The model under review builds one solid part; all positions refer to its coordinate system, in mm. Give positions to 0.01 mm unless a question says otherwise; leave off trailing zeros. Return JSON: item names as keys, results as strings. Group by question number.
from build123d import *

# Parameters (mm, degrees)
SKETCH1_W                      = 12
SKETCH1_H                      = 8
BOSS_EXTRUDE1_DEPTH            = 450
CBORE_FOR_M3_SHCS1_D           = 3.4
CBORE_FOR_M3_SHCS1_CBORE_D     = 6.5
CBORE_FOR_M3_SHCS1_CBORE_DEPTH = 4.5


with BuildPart() as part:
    # Sketch1 → Boss-Extrude1 (new body)
    with BuildSketch(Plane.XY):
        with Locations((6, 4)):
            Rectangle(SKETCH1_W, SKETCH1_H)
    extrude(amount=BOSS_EXTRUDE1_DEPTH)

    # CBORE for M3 SHCS1 (through all)
    with Locations(Plane(origin=(0, 8, 0), x_dir=(1, 0, 0), z_dir=(0, 1, 0))):
        with Locations((6, -440), (6, -415), (6, -390), (6, -365), (6, -340), (6, -315), (6, -290), (6, -265), (6, -240), (6, -215), (6, -190), (6, -165), (6, -140), (6, -115), (6, -90), (6, -65), (6, -40), (6, -15)):
            CounterBoreHole(CBORE_FOR_M3_SHCS1_D / 2, CBORE_FOR_M3_SHCS1_CBORE_D / 2, CBORE_FOR_M3_SHCS1_CBORE_DEPTH)


solid = part.part
Item 1: For P1, Ø2.5, axis at x = 6, z = 90, coming from the -Y side; P2, Ø3, axis at x = 5.5, z = 391, coming from the +Y side, all flat-tipped, find the tip position at first contact; note any pin that passes through.
Item 2: Take a section at A-A (y = 5.25). State how many separate pieces and enclosed holes the cut face has, then the cut area to 3 significant figures.
Item 3: For L1, parallel to X at y = 2.4, z = 65; L2, parallel to Y at x = 5, z = 118; L3, parallel to X at y = 5, z = 313.5, list the stretches that pass through material, from the lowest coordinate up. Write a range as from..to.
Check sheet entries:
{
 "1": {"P1": "passes through", "P2": "stops at y = 3.5"},
 "2": {"separate pieces": "1", "enclosed holes": "18", "area": "4,800 mm^2"},
 "3": {"L1": "x = 0..4.3, 7.7..12", "L2": "y = 0..3.5", "L3": "x = 0..3.12, 8.88..12"}
}
